Design review of the part built by this model. Coordinates are the model's own, in mm. Coordinates: 2 decimals unless noted, no trailing zeros. Write each loop counter-clockwise with the first axis right and the second up, starting at its lowest first coordinate (ties: lowest second). Pieces come first, ordered by that corner, then holes. Notation, with made-up numbers: (66.25, 38.5) - (95.25, 38.5) arc R9 ccw to (95.25, 51.5) - close; hole circle Ø7 at (61, 32). An arc over 180 degrees is marked (long way). Use a Markdown table: item, result.
from build123d import *

# Parameters (mm, degrees)
F1_DEPTH = 2.54
F4_DEPTH = 2.54
F5_W     = 25.4
F5_H     = 2.794
F6_DEPTH = 25.4


with BuildPart() as f1:
    # F0 (on Top) → F1 (new body)
    with BuildSketch(Plane.XY):
        with BuildLine():
            Line((206.375, -73.81875), (206.375, 73.81875))
            ThreePointArc((206.375, 73.81875), (196.145704, 98.514454), (171.45, 108.74375))
            Line((171.45, 108.74375), (-171.45, 108.74375))
            ThreePointArc((-171.45, 108.74375), (-196.145704, 98.514454), (-206.375, 73.81875))
            Line((-206.375, 73.81875), (-206.375, -73.81875))
            ThreePointArc((-206.375, -73.81875), (-196.145704, -98.514454), (-171.45, -108.74375))
            Line((-171.45, -108.74375), (171.45, -108.74375))
            ThreePointArc((171.45, -108.74375), (196.145704, -98.514454), (206.375, -73.81875))
        make_face()
        with BuildLine():
            ThreePointArc((187.325, -73.81875), (182.67532, -85.04407), (171.45, -89.69375))
            Line((171.45, -89.69375), (-171.45, -89.69375))
            ThreePointArc((-171.45, -89.69375), (-182.67532, -85.04407), (-187.325, -73.81875))
            Line((-187.325, -73.81875), (-187.325, 73.81875))
            ThreePointArc((-187.325, 73.81875), (-182.67532, 85.04407), (-171.45, 89.69375))
            Line((-171.45, 89.69375), (171.45, 89.69375))
            ThreePointArc((171.45, 89.69375), (182.67532, 85.04407), (187.325, 73.81875))
            Line((187.325, 73.81875), (187.325, -73.81875))
        make_face(mode=Mode.SUBTRACT)
    extrude(amount=F1_DEPTH)

    # F3 (on face) → F4 (join, through all)
    with BuildSketch(Plane.XY.offset(2.54)):
        with BuildLine():
            ThreePointArc((-186.176704, 79.746635), (-178.185192, 80.553942), (-177.377885, 88.545454))
            ThreePointArc((-177.377885, 88.545454), (-182.67532, 85.04407), (-186.176704, 79.746635))
        make_face()
        with BuildLine():
            ThreePointArc((186.176704, 79.746635), (182.67532, 85.04407), (177.377885, 88.545454))
            ThreePointArc((177.377885, 88.545454), (178.185192, 80.553942), (186.176704, 79.746635))
        make_face()
        with BuildLine():
            ThreePointArc((177.377885, -88.545454), (182.67532, -85.04407), (186.176704, -79.746635))
            ThreePointArc((186.176704, -79.746635), (178.185192, -80.553942), (177.377885, -88.545454))
        make_face()
        with BuildLine():
            ThreePointArc((-177.377885, -88.545454), (-178.185192, -80.553942), (-186.176704, -79.746635))
            ThreePointArc((-186.176704, -79.746635), (-182.67532, -85.04407), (-177.377885, -88.545454))
        make_face()
    extrude(amount=-F4_DEPTH)

    # F5 (on face) → F6 (cut)
    with BuildSketch(Plane.XY.offset(2.54)):
        with Locations((-107.315, 94.77375)):
            Rectangle(F5_W, F5_H)
        with Locations((138.7475, 94.77375)):
            Rectangle(F5_W, F5_H)
    extrude(amount=-F6_DEPTH, mode=Mode.SUBTRACT)


solid = f1.part
(1) Take a section at A-A on y = -50.5. Write out the cut boundary in (x, z) (3 decimals).
Determined:
| item | result |
|---|---|
| outline | (-206.375, 0) - (-187.325, 0) - (-187.325, 2.54) - (-206.375, 2.54) - close; (187.325, 0) - (206.375, 0) - (206.375, 2.54) - (187.325, 2.54) - close |
(2) For pin 1 (0.8 mm diameter, centred on y = 95.5, z = 1, fed in from +X); pin 2 (5 mm diameter, centred on x = 162.5, y = 86, fed in from +Z); pin 3 (1.3 mm diameter, centred on y = 95.5, z = 1, fed in from -X), all flat-tipped, find the tip position at first contact; note any pin that passes through.
Determined:
| item | result |
|---|---|
| pin 1 | x = 199.14 |
| pin 2 | through |
| pin 3 | x = -199.33 |
(3) Draft analysis for pull direction Y (two halves, no side actions). For faces 1 (the cylindrical face through (-178.27, 80.47, 1.29)), 2 (the cylindrical face through (-195.873, 98.784, 1.252)), 3 (the cylindrical face through (-196.416, -98.241, 1.252)), 4 (the cylindrical face through (-178.1, -80.64, 1.29)), state which applies: +Y half, -Y half, draft (parallel to the pull), parting line (faces both ways), or undercut.
Determined:
| item | result |
|---|---|
| face 1 | undercut |
| face 2 | +Y half |
| face 3 | -Y half |
| face 4 | undercut |
(4) Take a section at C-C on z = 1.2. State how many separate pieces and enclosed holes the cut face has, and give its area (3 significant figures).
Determined:
| item | result |
|---|---|
| separate pieces | 1 |
| enclosed holes | 3 |
| area | 21,800 mm2 |
(5) For L1, parallel to Y at x = -108, z = 0.45; L2, parallel to Y at x = 87.5, z = 1.7; L3, parallel to X at y = 1.5, z = 1.25 (3 decimals), list the stretches that pass through material, from the lowest coordinate up. Write a range as from..to.
Determined:
| item | result |
|---|---|
| L1 | -108.74..-89.69, 89.69..93.38, 96.17..108.74 |
| L2 | -108.74..-89.69, 89.69..108.74 |
| L3 | -206.375..-187.325, 187.325..206.375 |
(6) Take a section at D-D on x = 46. Write out the cut boundary in (y, z), and give its area (3 significant figures).
Determined:
| item | result |
|---|---|
| outline | (-108.74, 0) - (-89.69, 0) - (-89.69, 2.54) - (-108.74, 2.54) - close; (89.69, 0) - (108.74, 0) - (108.74, 2.54) - (89.69, 2.54) - close |
| area | 96.8 mm2 |
(7) Take a section at B-B on x = 134. Write out the cut boundary in (y, z).
Determined:
| item | result |
|---|---|
| outline | (-108.74, 0) - (-89.69, 0) - (-89.69, 2.54) - (-108.74, 2.54) - close; (89.69, 0) - (93.38, 0) - (93.38, 2.54) - (89.69, 2.54) - close; (96.17, 0) - (108.74, 0) - (108.74, 2.54) - (96.17, 2.54) - close |
